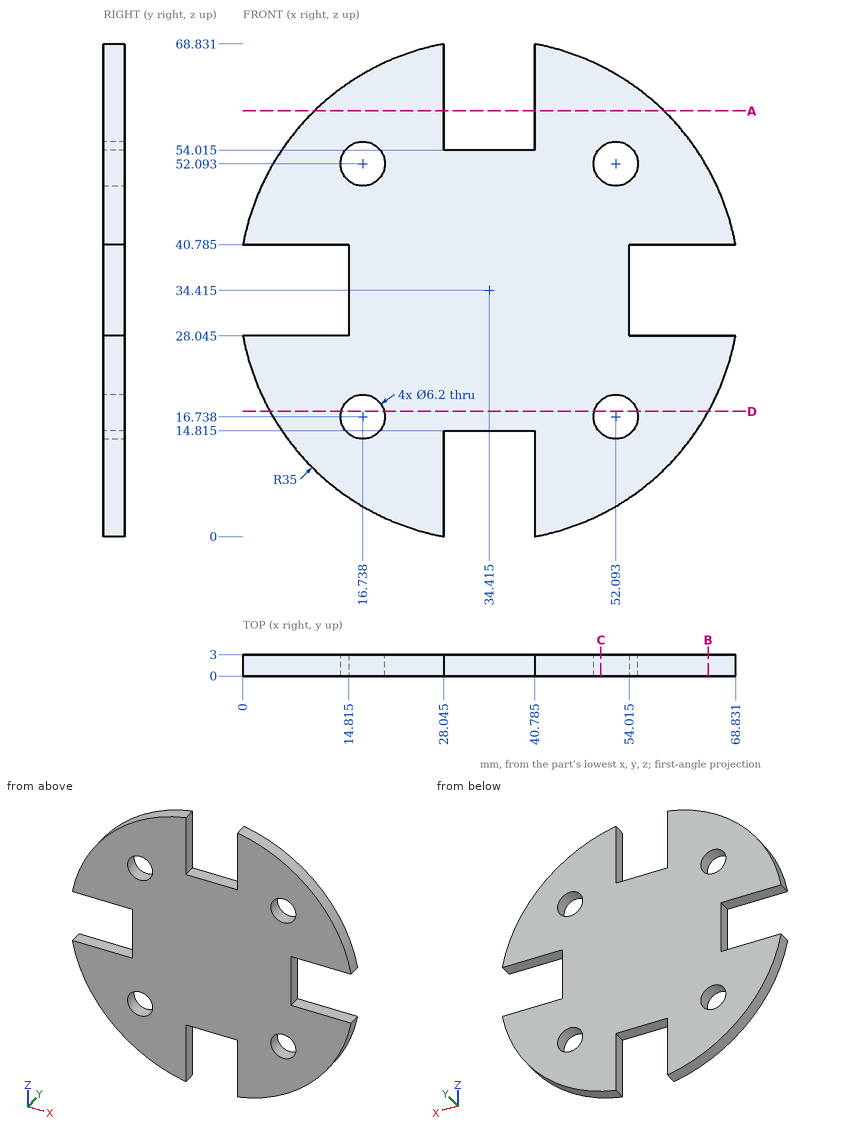
Here's the drawing with two shaded views (mm, measured from the low corner). I have some questions. Give positions to 0.01 mm unless a question says otherwise; leave off trailing zeros. Write each loop counter-clockwise with the first axis right and the second up, starting at its lowest first coordinate (ties: lowest second). Pieces come first, ordered by that corner, then holes. Notation, with made-up numbers: (70.5, 18) -> (95.5, 18) arc R7 cw to (95.5, 31) -> close; hole circle Ø1 at (40, 18). An arc over 180 degrees is marked (long way). Use one line per item in the form item = value. Start each with the question number.
1. Imagine slicing it at A-A on z = 59.5. List the corners of the cut face in (x, y) for me (1 decimal).
2. Imagine slicing it at D-D on z = 17.5. List the corners of the cut face in (x, y) for me (1 decimal).
3. Imagine slicing it at C-C on x = 50. List the corners of the cut face in (y, z) for me (1 decimal).
4. Will these pins go through, and if not, where does the flat tip stop? pin 1 Ø3.5 at (x, z) = (16.74, 16.74) entering from +Y; pin 2 Ø1.5 at (y, z) = (2, 25.5) entering from -X; pin 3 Ø0.9 at (y, z) = (1, 32.5) entering from -X (1 decimal); pin 4 Ø10 at (x, z) = (20, 20.5) entering from -Y.
5. Imagine slicing it at B-B on x = 65. List the corners of the cut face in (y, z) for me (1 decimal).
6. If I drill on L1, parallel to X at y = 0.9, z = 49.5 (1 decimal); L2, parallel to Z at x = 53.5, y = 2.95 (1 decimal); L3, parallel to Z at x = 19, y = 0.65 (1 decimal), over which ranges is the centre line in solid material (lowest first)?
Entries:
q1.outline = (10, 0) -> (28, 0) -> (28, 3) -> (10, 3) -> close; (40.8, 0) -> (58.8, 0) -> (58.8, 3) -> (40.8, 3) -> close
q2.outline = (3.8, 0) -> (13.7, 0) -> (13.7, 3) -> (3.8, 3) -> close; (19.7, 0) -> (49.1, 0) -> (49.1, 3) -> (19.7, 3) -> close; (55.1, 0) -> (65.1, 0) -> (65.1, 3) -> (55.1, 3) -> close
q3.outline = (0, 3.1) -> (3, 3.1) -> (3, 14.5) -> (0, 14.5) -> close; (0, 19) -> (3, 19) -> (3, 49.8) -> (0, 49.8) -> close; (0, 54.4) -> (3, 54.4) -> (3, 65.8) -> (0, 65.8) -> close
q4.pin_1 = through
q4.pin_2 = 0.38
q4.pin_3 = 14.8
q4.pin_4 = 0
q5.outline = (0, 17.4) -> (3, 17.4) -> (3, 28) -> (0, 28) -> close; (0, 40.8) -> (3, 40.8) -> (3, 51.4) -> (0, 51.4) -> close
q6.L1 = 2.8 to 15, 18.4 to 50.4, 53.8 to 66
q6.L2 = 5.1 to 14, 19.5 to 49.3, 54.9 to 63.8
q6.L3 = 3 to 14.6, 18.9 to 50, 54.2 to 65.8
